Can you work these out from the model? Positions are in its coordinate system, mm. Give positions to 0.01 mm unless a question says otherwise; leave off trailing zeros. Loops run counter-clockwise (first coordinate to the right, second up) from the corner with the lowest first, then second, coordinate; pieces in that order, holes last. Notation, with made-up numbers: M -9.5,16 L 8.5,16 A17 cw 8.5,37 Z; hole C -0.5,74.25 d2. An arc over 180 degrees is marked long. Use CSV: the item, a comma, the result in double quotes.
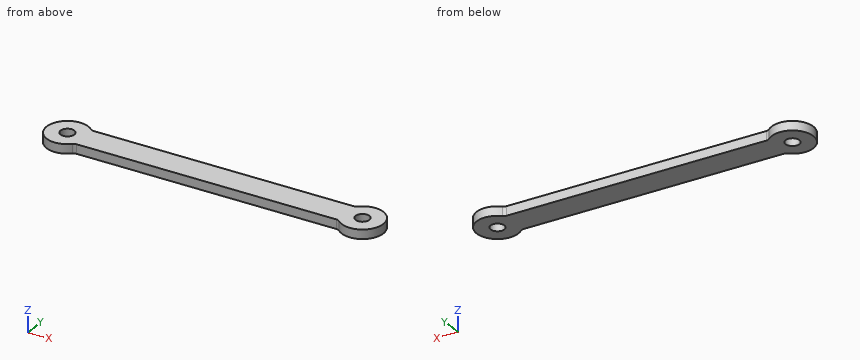
from build123d import *

# Parameters (mm, degrees)
F0_R     = 15
F1_DEPTH = 20


with BuildPart() as f1:
    # F0 (on Top) → F1 (new body)
    with BuildSketch(Plane.XY):
        with BuildLine():
            ThreePointArc((344.388068, -30), (348.080813, -30.706796), (351.251554, -32.727273))
            ThreePointArc((351.251554, -32.727273), (427.13724, 0), (351.251554, 32.727273))
            ThreePointArc((351.251554, 32.727273), (348.080813, 30.706796), (344.388068, 30))
            Line((344.388068, 30), (-214.609888, 30))
            ThreePointArc((-214.609888, 30), (-218.302632, 30.706796), (-221.473374, 32.727273))
            ThreePointArc((-221.473374, 32.727273), (-297.35906, 0), (-221.473374, -32.727273))
            ThreePointArc((-221.473374, -32.727273), (-218.302632, -30.706796), (-214.609888, -30))
            Line((-214.609888, -30), (344.388068, -30))
        make_face()
        with Locations((-252.35906, 0)):
            Circle(F0_R, mode=Mode.SUBTRACT)
        with Locations((382.13724, 0)):
            Circle(F0_R, mode=Mode.SUBTRACT)
    extrude(amount=F1_DEPTH)


solid = f1.part
Q1. I'm going to push flat-ended pins straight in: P1, Ø1, axis at y = -17.5, z = 8.5, coming from the -X side; P2, Ø1, axis at x = 338, y = -25.5, coming from the -Z side; P3, Ø1.5, axis at y = 1, z = 9, coming from the -X side; P4, Ø12, axis at y = -15.5, z = 11, coming from the -X side. Where does each tip first touch, or does it pass through?
Model answer:
P1,"x = -294.02"
P2,"z = 0"
P3,"x = -297.36"
P4,"x = -296.34"
Q2. Please list where these lines run through material, in increasing order: L1, parallel to X at y = -2, z = 16.25; L2, parallel to X at y = -4, z = 8.5; L3, parallel to Y at x = 299, z = 8.5. Write a range as from..to.
Model answer:
L1,"-297.31..-267.23, -237.49..367.27, 397..427.09"
L2,"-297.18..-266.82, -237.9..367.68, 396.59..426.96"
L3,"-30..30"
Q3. I want a section at A-A, the plane y = 0. Please give me the cut outline in (x, z).
Model answer:
outline,"M -297.36,0 L -267.36,0 L -267.36,20 L -297.36,20 Z; M -237.36,0 L 367.14,0 L 367.14,20 L -237.36,20 Z; M 397.14,0 L 427.14,0 L 427.14,20 L 397.14,20 Z"
Q4. I want a section at B-B, the plane z = 6.5. Please give me the cut outline in (x, y), then the cut area to 3 significant figures.
Model answer:
outline,"M -221.47,-32.73 A10 cw -214.61,-30 L 344.39,-30 A10 cw 351.25,-32.73 A45 ccw long 351.25,32.73 A10 cw 344.39,30 L -214.61,30 A10 cw -221.47,32.73 A45 ccw long Z; hole C -252.36,0 d30; hole C 382.14,0 d30"
area,"44,400 mm2"
Q5. I want a section at C-C, the plane x = -178.5. Please give me the cut outline in (y, z), then the cut area to 3 significant figures.
Model answer:
outline,"M -30,0 L 30,0 L 30,20 L -30,20 Z"
area,"1,200 mm2"
